Read the model definition and answer for the solid it produces. Units are mm, in the model's axes. Face numbers are marked on the shaded views. A direction names the side the tool comes from. Round coordinates to 2 decimals unless told otherwise and drop trailing zeros. Order: outer loops, then holes, each group sorted by start corner. A loop starts at its lowest first (then second) coordinate and runs counter-clockwise, first axis right, second up. Notation, with made-up numbers: (-15.75, -5) - (-4.75, -5) arc R24 cw to (-4.75, 8) - close; hole circle Ø1 at (5.25, -22). An arc over 180 degrees is marked (long way). Answer as a JSON object with one key per item and string values. Group by question number.
Q1. A cutting plane is placed at A-A on y = 2.3. Determine the outline of the cut face in (x, z), and give its area (3 significant figures).
Q2. The mould has two halves that part along Z. Classify the marked faces 1, 2 and 3: pulls with the +Z half, pulls with the -Z half, needs draft (parallel to the pull), parting line crosses it, or undercut.
Q3. Given pin 1 Ø1.8 at (x, z) = (3, -2) entering from -Y; pin 2 Ø1.5 at (y, z) = (2, -14) entering from -X, each flat-ended and moving along its own axis, determine where each tip first touches the part or whether it passes through.
Q4. A tool of negligible diameter and unlimited length cuts with its end or side. For the marked faces 4 and 5, from which of +Z, -Z, +X, -X, +Y, -Y can it reach the whole face along a straight path? Write none if from no direction.
Q5. Consider line 1 (Z direction, x = 17.5, y = 3.2); line 2 (X direction, y = 2.65, z = -33); line 3 (Z direction, x = 2.5, y = 1.95). Determine where each line is inside the solid, lowest interval first.
Q6. A cutting plane is placed at D-D on x = 23.5. Determine the outline of the cut face in (y, z).
Q7. A cutting plane is placed at B-B on x = 19. Determine the outline of the cut face in (y, z), and give its area (3 significant figures).
Q8. A cutting plane is placed at C-C on z = -25.5. Determine the outline of the cut face in (x, y), and give its area (3 significant figures).
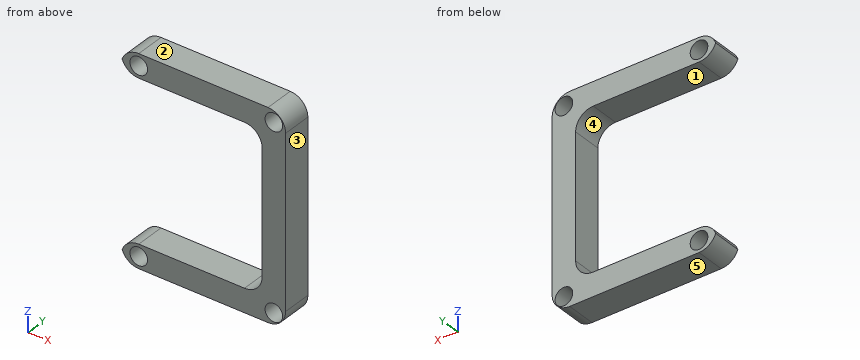
```python
from build123d import *

# Parameters (mm, degrees)
SKETCH1_R           = 1.5
BOSS_EXTRUDE1_DEPTH = 5
FILLET2_R           = 3


with BuildPart() as part:
    # Sketch1 → Boss-Extrude1 (new body)
    with BuildSketch(Plane(origin=(0, 0, 0), x_dir=(1, 0, 0), z_dir=(0, 1, 0))):
        Polygon((0, 31), (0, 35), (28, 35), (28, 0), (0, 0), (0, 4), (24, 4), (24, 31), align=None)
        with Locations(Location((26, 2, 0), (0, 0, 270))):
            Circle(SKETCH1_R, mode=Mode.SUBTRACT)
        with Locations(Location((26, 33, 0), (0, 0, 270))):
            Circle(SKETCH1_R, mode=Mode.SUBTRACT)
        with Locations(Location((3, 33, 0), (0, 0, 270))):
            Circle(SKETCH1_R, mode=Mode.SUBTRACT)
        with Locations(Location((3, 2, 0), (0, 0, 270))):
            Circle(SKETCH1_R, mode=Mode.SUBTRACT)
    extrude(amount=BOSS_EXTRUDE1_DEPTH)

    # Fillet2
    # the kernel refuses this fillet: 3 mm, written as the material it adds along each edge
    with BuildSketch(Plane(origin=(24, 0, -31), x_dir=(0, 0, 1), z_dir=(0, 1, 0)), Plane(origin=(24, 0, -4), x_dir=(-1, 0, 0), z_dir=(0, 1, 0))) as fillet2_piece_1:
        with BuildLine():
            CenterArc((FILLET2_R, -FILLET2_R), FILLET2_R, 90, 90)
            Line((0, -FILLET2_R), (0, 0))
            Line((0, 0), (FILLET2_R, 0))
        make_face()
    extrude(amount=5)
    # the kernel refuses this fillet: 3 mm, written as the material it takes off along each edge
    with BuildSketch(Plane(origin=(28, -7.5, -35), x_dir=(-1, 0, 0), z_dir=(0, 1, 0)), Plane(origin=(0, -7.5, -35), x_dir=(0, 0, 1), z_dir=(0, 1, 0)), Plane(origin=(0, -7.5, -4), x_dir=(0, 0, 1), z_dir=(0, 1, 0)), Plane(origin=(0, -7.5, 0), x_dir=(1, 0, 0), z_dir=(0, 1, 0)), Plane(origin=(28, -7.5, 0), x_dir=(0, 0, -1), z_dir=(0, 1, 0))) as fillet2_2_piece_1:
        with BuildLine():
            CenterArc((FILLET2_R, FILLET2_R), FILLET2_R, 180, 90)
            Line((0, FILLET2_R), (0, 0))
            Line((0, 0), (FILLET2_R, 0))
        make_face()
    extrude(amount=20, mode=Mode.SUBTRACT)
    with BuildSketch(Plane(origin=(0, -7.5, -31), x_dir=(0, 0, -1), z_dir=(0, 1, 0))) as fillet2_2_piece_2:
        with BuildLine():
            CenterArc((FILLET2_R, -FILLET2_R), FILLET2_R, 90, 90)
            Line((0, -FILLET2_R), (0, 0))
            Line((0, 0), (FILLET2_R, 0))
        make_face()
    extrude(amount=20, mode=Mode.SUBTRACT)


solid = part.part
```
Result set:
{
 "1": {"outline": "(0.17, -33) arc R3 ccw to (3, -35) - (25, -35) arc R3 ccw to (28, -32) - (28, -3) arc R3 ccw to (25, 0) - (3, 0) arc R3 ccw to (0.17, -2) arc R3 ccw to (3, -4) - (21, -4) arc R3 cw to (24, -7) - (24, -28) arc R3 cw to (21, -31) - (3, -31) arc R3 ccw to start; hole circle Ø3 at (3, -33); hole circle Ø3 at (3, -2); hole circle Ø3 at (26, -33); hole circle Ø3 at (26, -2)", "area": "296 mm²"},
 "2": {"face 1": "undercut", "face 2": "pulls with the +Z half", "face 3": "needs draft"},
 "3": {"pin 1": "passes through", "pin 2": "stops at x = 24"},
 "4": {"face 4": "-X, +Y, -Y", "face 5": "-Z, +X, -X, +Y, -Y"},
 "5": {"line 1": "z = -35 to -31, -4 to 0", "line 2": "x = 0.17 to 1.5, 4.5 to 24.5, 27.5 to 27.83", "line 3": "z = -34.96 to -34.41, -31.59 to -31.04, -3.96 to -3.41, -0.59 to -0.04"},
 "6": {"outline": "(0, -35) - (5, -35) - (5, -29.66) - (0, -29.66) - close; (0, -5.34) - (5, -5.34) - (5, 0) - (0, 0) - close"},
 "7": {"outline": "(0, -35) - (5, -35) - (5, -31) - (0, -31) - close; (0, -4) - (5, -4) - (5, 0) - (0, 0) - close", "area": "40.0 mm²"},
 "8": {"outline": "(24, 0) - (28, 0) - (28, 5) - (24, 5) - close", "area": "20.0 mm²"}
}
